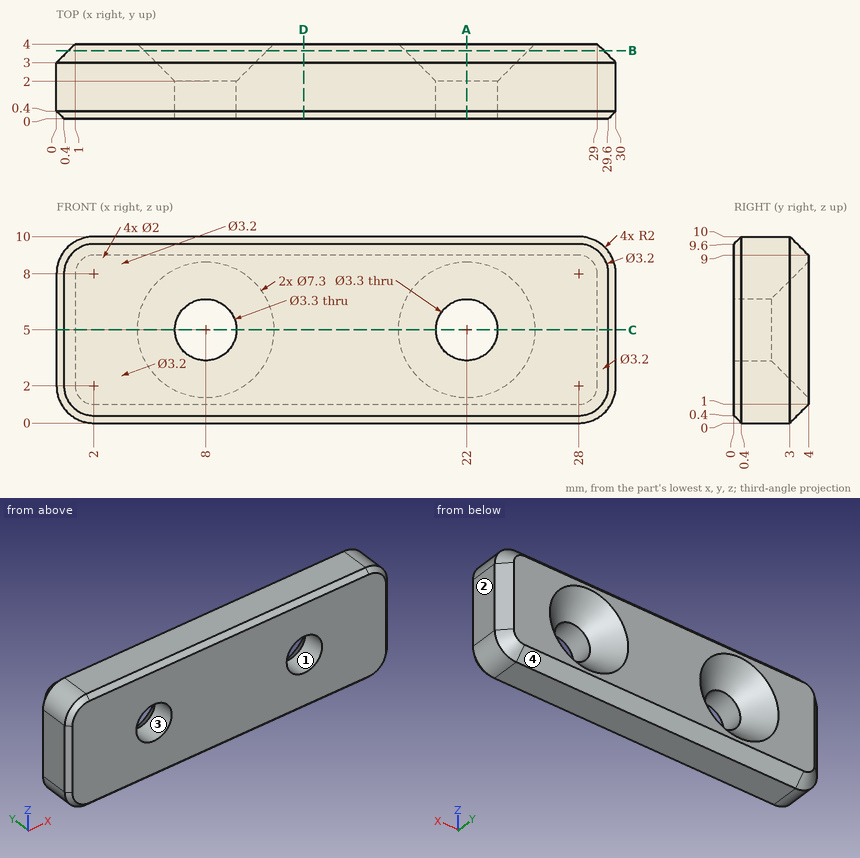
Answer from the drawing. Dimensions are ordinates in mm from the lowest x, y and z of the part. Round coordinates to 2 decimals unless told otherwise and drop trailing zeros. Loops run counter-clockwise (first coordinate to the right, second up) from the corner with the lowest first, then second, coordinate; pieces in that order, holes last. Notation, with made-up numbers: (67, 67) - (99, 67) arc R22 ccw to (99, 94) - close; hole circle Ø1 at (9.5, 59). An arc over 180 degrees is marked (long way). Return JSON: item names as keys, results as strings. Group by question number.
1. The part is cut by section B-B on y = 3.65. Determine the outline of the cut face in (x, z), then the cut area to 3 significant figures.
2. The part is cut by section D-D on x = 13.25. Determine the outline of the cut face in (y, z).
3. The mould has two halves that part along X. Classify the marked faces 1, 2, 3 and 4: pulls with the +X half, pulls with the -X half, needs draft (parallel to the pull), parting line crosses it, or undercut.
4. The part is cut by section C-C on z = 5. Determine the outline of the cut face in (x, y).
5. The part is cut by section A-A on x = 22. Determine the outline of the cut face in (y, z), then the cut area to 3 significant figures.
6. Consider probe 1 along X at (y, z) = (0.5, 5); probe 2 along X at (y, z) = (1.55, 6); probe 3 along Z at (x, y) = (23.25, 1.7). Determine where each line is inside the solid, lowest interval first.
Resolved:
{
 "1": {"outline": "(0.65, 2) arc R1.35 ccw to (2, 0.65) - (28, 0.65) arc R1.35 ccw to (29.35, 2) - (29.35, 8) arc R1.35 ccw to (28, 9.35) - (2, 9.35) arc R1.35 ccw to (0.65, 8) - close; hole circle Ø6.6 at (8, 5); hole circle Ø6.6 at (22, 5)", "area": "180 mm²"},
 "2": {"outline": "(0, 0.4) - (0.4, 0) - (3, 0) - (4, 1) - (4, 9) - (3, 10) - (0.4, 10) - (0, 9.6) - close"},
 "3": {"face 1": "undercut", "face 2": "pulls with the +X half", "face 3": "undercut", "face 4": "needs draft"},
 "4": {"outline": "(0, 0.4) - (0.4, 0) - (6.35, 0) - (6.35, 2) - (4.35, 4) - (1, 4) - (0, 3) - close; (9.65, 0) - (20.35, 0) - (20.35, 2) - (18.35, 4) - (11.65, 4) - (9.65, 2) - close; (23.65, 0) - (29.6, 0) - (30, 0.4) - (30, 3) - (29, 4) - (25.65, 4) - (23.65, 2) - close"},
 "5": {"outline": "(0, 0.4) - (0.4, 0) - (3, 0) - (4, 1) - (4, 1.35) - (2, 3.35) - (0, 3.35) - close; (0, 6.65) - (2, 6.65) - (4, 8.65) - (4, 9) - (3, 10) - (0.4, 10) - (0, 9.6) - close", "area": "21.6 mm²"},
 "6": {"probe 1": "x = 0 to 6.35, 9.65 to 20.35, 23.65 to 30", "probe 2": "x = 0 to 6.69, 9.31 to 20.69, 23.31 to 30", "probe 3": "z = 0 to 3.92, 6.08 to 10"}
}
